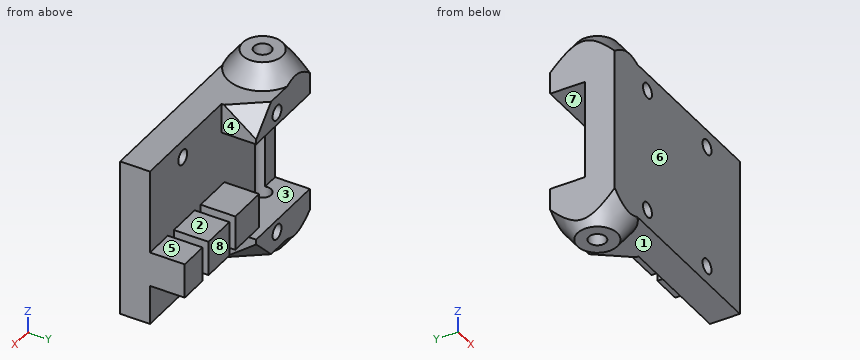
from build123d import *

# Parameters (mm, degrees)
SKETCH1_W           = 42
SKETCH1_H           = 32
BOSS_EXTRUDE1_DEPTH = 6
SKETCH4_W           = 18
SKETCH4_H           = 6
SKETCH4_W_2         = 7
SKETCH4_H_2         = 7
SKETCH4_W_3         = 6
SKETCH4_W_4         = 8
BOSS_EXTRUDE2_DEPTH = 7
SKETCH9_R           = 1.725
CUT_EXTRUDE2_DEPTH  = 61.301326685
SKETCH10_W          = 6
SKETCH10_H          = 13
BOSS_EXTRUDE5_DEPTH = 11
SKETCH5_R           = 1.5
CUT_EXTRUDE3_DEPTH  = 57.824290581
CHAMFER1_START      = 14.286772629
CHAMFER1_DEPTH      = 3.105820136
CHAMFER2_START      = -5.671483031
CHAMFER2_DEPTH      = 11.890532792


with BuildPart() as part:
    # Sketch1 → Boss-Extrude1 (new body)
    with BuildSketch(Plane(origin=(0, 0, 0), x_dir=(1, 0, 0), z_dir=(0, 1, 0))):
        with Locations((21, 16)):
            Rectangle(SKETCH1_W, SKETCH1_H)
    extrude(amount=BOSS_EXTRUDE1_DEPTH)

    # Sketch3 → Revolve2 (revolve)
    with BuildSketch(Plane(origin=(0, 6.5, 0), x_dir=(1, 0, 0), z_dir=(0, 1, 0)), mode=Mode.PRIVATE) as revolve2_sk:
        Polygon((5, 28), (-5, 28), (1, 36), (5, 36), align=None)
        Polygon((5, -4), (5, 4), (-5, 4), (1, -4), align=None)
    revolve(revolve2_sk.sketch.rotate(Axis((5, 6.5, -28), (0, 0, 1)), 177.134016017), axis=Axis((5, 6.5, -28), (0, 0, 1)))

    # Sketch4 → Boss-Extrude2 (add)
    with BuildSketch(Plane(origin=(0, 6, 0), x_dir=(1, 0, 0), z_dir=(0, 1, 0))):
        with Locations((9, 29)):
            Rectangle(SKETCH4_W, SKETCH4_H)
        with Locations((30.5, 20.5)):
            Rectangle(SKETCH4_W_2, SKETCH4_H_2)
        with Locations((39, 20.5)):
            Rectangle(SKETCH4_W_3, SKETCH4_H_2)
        with Locations((21, 20.5)):
            Rectangle(SKETCH4_W_4, SKETCH4_H_2)
        with Locations((9, 3)):
            Rectangle(SKETCH4_W, SKETCH4_H)
    extrude(amount=BOSS_EXTRUDE2_DEPTH)

    # Sketch7 → Cut-Revolve1 (revolve, cut)
    with BuildSketch(Plane(origin=(0, 6.5, 0), x_dir=(1, 0, 0), z_dir=(0, 1, 0))):
        Polygon((-5, 4), (1, -4), (-5, -4), align=None)
        Polygon((-5, 28), (1, 36), (-5, 36), align=None)
    revolve(axis=Axis((5, 6.5, -36), (0, 0, 1)), mode=Mode.SUBTRACT)

    # Sketch9 → Cut-Extrude2 (cut, through all)
    with BuildSketch(Plane.XY.offset(4)):
        with Locations((5, 6.5)):
            Circle(SKETCH9_R)
        Polygon((18, 13), (0, 13), (0, 0), (18, 0), (18, -5), (-7, -5), (-7, 18), (18, 18), align=None)
    extrude(amount=-CUT_EXTRUDE2_DEPTH, mode=Mode.SUBTRACT)

    # Sketch10 → Boss-Extrude5 (add)
    with BuildSketch(Plane(origin=(18, 0, 0), x_dir=(0, 0, -1), z_dir=(1, 0, 0))):
        with Locations((3, 6.5)):
            Rectangle(SKETCH10_W, SKETCH10_H)
        with Locations((29, 6.5)):
            Rectangle(SKETCH10_W, SKETCH10_H)
    extrude(amount=-BOSS_EXTRUDE5_DEPTH)

    # Sketch5 → Cut-Extrude3 (cut, through all)
    with BuildSketch(Plane(origin=(0, 0, 0), x_dir=(1, 0, 0), z_dir=(0, 1, 0))):
        with Locations(Location((11, 28.5, 0), (0, 0, 270))):
            Circle(SKETCH5_R)
        with Locations(Location((31, 28.5, 0), (0, 0, 90))):
            Circle(SKETCH5_R)
        with Locations(Location((31, 3.5, 0), (0, 0, 90))):
            Circle(SKETCH5_R)
        with Locations(Location((11, 3.5, 0), (0, 0, 270))):
            Circle(SKETCH5_R)
    extrude(amount=CUT_EXTRUDE3_DEPTH, mode=Mode.SUBTRACT)

    # Chamfer1: read off the stored shape, not the designer's step
    # Chamfer1 outline → Chamfer1 (cut)
    with BuildSketch(Plane(origin=(0, 0, 0), x_dir=(0.7836805797909963, -0.3787303917205566, -0.49234950923672277), z_dir=(0.6211640273377459, 0.4778184825674969, 0.6211640273377449)).offset(CHAMFER1_START)):
        Polygon((11.64450289, 5.152055929), (11.64450289, 13.352665663), (5.264352445, 10.304111858), align=None)
    extrude(amount=CHAMFER1_DEPTH, mode=Mode.SUBTRACT)

    # Chamfer2: read off the stored shape, not the designer's step
    # Chamfer2 outline → Chamfer2 (cut)
    with BuildSketch(Plane(origin=(0, 0, 0), x_dir=(0.7926239891045996, 0.6097107608496931, 0), z_dir=(0.6097107608496931, -0.7926239891045995, 0)).offset(CHAMFER2_START)):
        Polygon((22.193471695, -27), (18.230351749, -32), (24, -32), (24, -25), (23.778719673, -25), align=None)
    extrude(amount=CHAMFER2_DEPTH, mode=Mode.SUBTRACT)


solid = part.part
The listing builds one solid part. Answer for the finished solid, in the listing's coordinates (mm). Face numbers are marked on the shaded views. A direction names the side the tool comes from. Give positions to 0.01 mm unless a question says otherwise; leave off trailing zeros. Loops run counter-clockwise (first coordinate to the right, second up) from the corner with the lowest first, then second, coordinate; pieces in that order, holes last. Notation, with made-up numbers: (80, 12.25) - (124, 12.25) arc R21 cw to (124, 47.25) - close; hole circle Ø5 at (-18.5, 19). An arc over 180 degrees is marked (long way). Use one line per item in the form item = value.
1. Find the intervals of material crossed by line 1 along Z through (x, y) = (31, 3.1); line 2 along X through (y, z) = (1.2, -28.5); line 3 along X through (y, z) = (6.5, -28.5) (3 decimals), in increasing order. Write a range as [from, to].
Calculated:
line_1 = [-32, -30], [-27, -5], [-2, 0]
line_2 = [0, 9.5], [12.5, 29.5], [32.5, 42]
line_3 = [0, 3.275], [6.725, 9.5], [12.5, 18]
2. The mould has two halves that part along Z. Classify the marked faces 1, 2 and 3: pulls with the +Z half, pulls with the -Z half, needs draft (parallel to the pull), parting line crosses it, or undercut.
Calculated:
face_1 = pulls with the -Z half
face_2 = pulls with the +Z half
face_3 = undercut
3. Section D-D on z = -23 is taken. Give the vertices of the cut face in (x, y) (3 decimals).
Calculated:
outline = (0, 0) - (42, 0) - (42, 13) - (36, 13) - (36, 6) - (34, 6) - (34, 13) - (27, 13) - (27, 6) - (25, 6) - (25, 13) - (17, 13) - (17, 6) - (6.651, 6) arc R1.725 cw to (3.349, 6) - (0, 6) - close
4. Section A-A on z = -28.5 is taken. Give the vertices of the cut face in (x, y) (3 decimals).
Calculated:
outline = (0, 0) - (9.5, 0) - (9.5, 13) - (0, 13) - close; (12.5, 0) - (29.5, 0) - (29.5, 6) - (18, 6) - (18, 11.05) - (16.5, 13) - (12.5, 13) - close; (32.5, 0) - (42, 0) - (42, 6) - (32.5, 6) - close; hole circle Ø3.45 at (5, 6.5)
5. Section B-B on x = 5 is taken. Give the vertices of the cut face in (y, z) (3 decimals).
Calculated:
outline = (0, -32.667) - (2.5, -36) - (4.775, -36) - (4.775, 4) - (2.5, 4) - (0, 0.667) - close; (8.225, -36) - (10.5, -36) - (13, -32.667) - (13, -26) - (8.225, -26) - close; (8.225, -6) - (13, -6) - (13, 0.667) - (10.5, 4) - (8.225, 4) - close
6. Given pin 1 Ø3 at (y, z) = (11, -7) entering from +X; pin 2 Ø5 at (x, z) = (31, -3.5) entering from +Y; pin 3 Ø5.5 at (y, z) = (8.5, -20.5) entering from -X; pin 4 Ø1 at (x, y) = (13.5, 10) entering from +Z, each flat-ended and moving along its own axis, determine where each tip first touches the part or whether it passes through.
Calculated:
pin_1 = 18
pin_2 = 6
pin_3 = 0
pin_4 = 0
7. Section C-C on x = 22.5 is taken. Give the vertices of the cut face in (y, z), then the cut area to 3 significant figures.
Calculated:
outline = (0, -32) - (6, -32) - (6, -24) - (13, -24) - (13, -17) - (6, -17) - (6, 0) - (0, 0) - close
area = 241 mm^2
8. Which of the six approach directions +Z, -Z, +X, -X, +Y, -Y give full straight-line access (tool end or side, diameter ignored) to the marked faces 4, 5, 6, 7 and 8?
Calculated:
face_4 = +Z, +X, +Y
face_5 = +Z, +X, -X, +Y
face_6 = +Z, -Z, +X, -X, -Y
face_7 = +X, -X, +Y
face_8 = +Z, -Z, +X, -X, +Y
